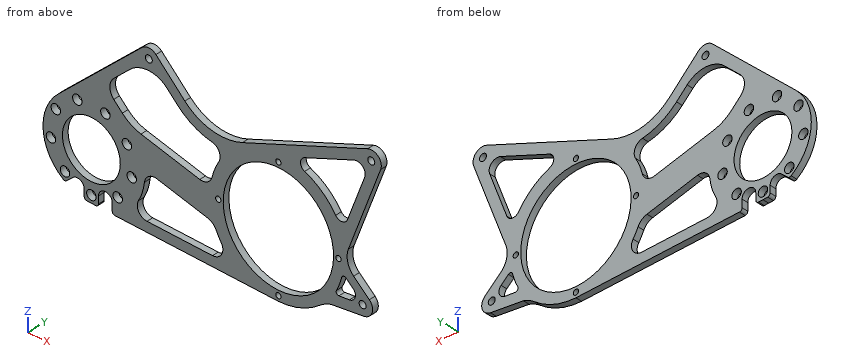
from build123d import *

# Parameters (mm, degrees)
MASTER_SKETCH_R       = 52.451
MASTER_SKETCH_R_2     = 9.525
MASTER_SKETCH_R_3     = 45.974
MASTER_SKETCH_R_4     = 27.4955
MASTER_SKETCH_R_5     = 6.5
BOSS_EXTRUDE2_DEPTH   = 3.048
F_5_0MM_DOWEL_HOLE1_D = 5
CIRPATTERN4_COUNT     = 4
M6_CLEARANCE_HOLE4_D  = 6.6
M8_CLEARANCE_HOLE1_D  = 9
CIRPATTERN3_COUNT     = 9
CUT_EXTRUDE2_DEPTH    = 284.854467488
CUT_EXTRUDE3_DEPTH    = 284.854467488
FILLET1_R             = 2.54


with BuildPart() as part:
    # Master Sketch → Boss-Extrude2 (new, symmetric)
    # profile 1 of 5: a face of its own
    with BuildSketch(Plane(origin=(0, 0, 0), x_dir=(1, 0, 0), z_dir=(0, 1, 0))):
        with BuildLine():
            ThreePointArc((-8.636, 127), (-36.396097826, 84.787887478), (-86.152093601, 93.552952189))
            Line((-86.152093601, 93.552952189), (-6.534964144, 18.470363023))
            ThreePointArc((-6.534964144, 18.470363023), (-3.773598517, 34.145603423), (9.525, 25.4))
            ThreePointArc((9.525, 25.4), (8.799952547, 21.754940307), (6.735192091, 18.664807909))
            Line((6.735192091, 18.664807909), (34.255961574, 46.185577392))
            ThreePointArc((34.255961574, 46.185577392), (59.945142207, 60.02346539), (89.010077776, 57.44457682))
            Line((89.010077776, 57.44457682), (207.987004211, 9.951947906))
            ThreePointArc((207.987004211, 9.951947906), (204.851852042, 25.601533276), (220.43444462, 22.148779315))
            Line((220.43444462, 22.148779315), (189.716874265, 103.891447497))
            ThreePointArc((189.716874265, 103.891447497), (189.0323732, 115.067445458), (194.744907427, 124.697524629))
            Line((194.744907427, 124.697524629), (209.652959731, 138.231042786))
            ThreePointArc((209.652959731, 138.231042786), (194.181291125, 142.373055798), (204.353700493, 154.744429565))
            Line((204.353700493, 154.744429565), (173.100049306, 158.387997533))
            ThreePointArc((173.100049306, 158.387997533), (167.382597042, 160.73155253), (162.227355528, 164.138163067))
            ThreePointArc((162.227355528, 164.138163067), (143.898999717, 174.415513345), (123.19, 177.9778))
            Line((123.19, 177.9778), (-54.61, 172.974))
            ThreePointArc((-54.61, 172.974), (-22.101472842, 159.508527158), (-8.636, 127))
        make_face()
        with Locations(Location((123.19, 116.0018, 0), (0, 0, 90))):
            Circle(MASTER_SKETCH_R, mode=Mode.SUBTRACT)
    # profile 2 of 5: a face of its own
    with BuildSketch(Plane(origin=(0, 0, 0), x_dir=(1, 0, 0), z_dir=(0, 1, 0))):
        with Locations((0, 25.4)):
            Circle(MASTER_SKETCH_R_2)
    # profile 3 of 5: a face of its own
    with BuildSketch(Plane(origin=(0, 0, 0), x_dir=(1, 0, 0), z_dir=(0, 1, 0))):
        with Locations((211.518208908, 18.79820239)):
            Circle(MASTER_SKETCH_R_2)
    # profile 4 of 5: a face of its own
    with BuildSketch(Plane(origin=(0, 0, 0), x_dir=(1, 0, 0), z_dir=(0, 1, 0))):
        with Locations((203.2507406, 145.283504427)):
            Circle(MASTER_SKETCH_R_2)
    # profile 5 of 5: a face of its own
    with BuildSketch(Plane(origin=(0, 0, 0), x_dir=(1, 0, 0), z_dir=(0, 1, 0))):
        with Locations((-54.61, 127)):
            Circle(MASTER_SKETCH_R_3)
        with Locations(Location((-54.61, 127, 0), (0, 0, 90))):
            Circle(MASTER_SKETCH_R_4, mode=Mode.SUBTRACT)
        with Locations(Location((-67.94878559, 163.648012211, 0), (0, 0, 90))):
            Circle(MASTER_SKETCH_R_5, mode=Mode.SUBTRACT)
        with Locations(Location((-41.27121441, 163.648012211, 0), (0, 0, 90))):
            Circle(MASTER_SKETCH_R_5, mode=Mode.SUBTRACT)
    extrude(amount=BOSS_EXTRUDE2_DEPTH, both=True)

    # Ø5.0mm Dowel Hole1 (through all)
    with Locations(Plane(origin=(0, 3.048, 0), x_dir=(1, 0, 0), z_dir=(0, 1, 0))):
        with Locations((123.19, 173.1518)):
            f_5_0mm_dowel_hole1 = Hole(F_5_0MM_DOWEL_HOLE1_D / 2)

    # CirPattern4: Ø5.0mm Dowel Hole1 ×4 about axis
    cirpattern4_axis = Axis((123.19, 0, -116.0018), (0, 1, 0))
    for i in range(1, CIRPATTERN4_COUNT):
        add(f_5_0mm_dowel_hole1.rotate(cirpattern4_axis, i * 360 / CIRPATTERN4_COUNT), mode=Mode.SUBTRACT)

    # M6 Clearance Hole4 (through all)
    with Locations(Plane(origin=(0, 3.048, 0), x_dir=(1, 0, 0), z_dir=(0, 1, 0))):
        with Locations((203.2507406, 145.283504427), (211.518208908, 18.79820239), (0, 25.4)):
            Hole(M6_CLEARANCE_HOLE4_D / 2)

    # M8 Clearance Hole1 (through all)
    with Locations(Plane(origin=(0, 3.048, 0), x_dir=(1, 0, 0), z_dir=(0, 1, 0))):
        with Locations((-54.61, 166)):
            m8_clearance_hole1 = Hole(M8_CLEARANCE_HOLE1_D / 2)

    # CirPattern3: M8 Clearance Hole1 ×9 about axis
    cirpattern3_axis = Axis((-54.61, 0, -127), (0, 1, 0))
    for i in range(1, CIRPATTERN3_COUNT):
        add(m8_clearance_hole1.rotate(cirpattern3_axis, i * 360 / CIRPATTERN3_COUNT), mode=Mode.SUBTRACT)

    # Topology 3 → Cut-Extrude2 (cut, through all)
    with BuildSketch(Plane(origin=(0, 3.048, 0), x_dir=(1, 0, 0), z_dir=(0, 1, 0))):
        with BuildLine():
            ThreePointArc((-17.945313453, 42.323250142), (-0.146601343, 35.405008389), (17.44176984, 42.84176984))
            Line((17.44176984, 42.84176984), (27.520769483, 52.920769483))
            ThreePointArc((27.520769483, 52.920769483), (42.409632623, 63.819008448), (59.896219631, 69.707058463))
            ThreePointArc((59.896219631, 69.707058463), (66.885503662, 75.024623751), (66.553177874, 83.800508404))
            ThreePointArc((66.553177874, 83.800508404), (62.745475764, 91.688999032), (60.030376503, 100.016970919))
            ThreePointArc((60.030376503, 100.016970919), (55.6852269, 105.854731176), (48.48636159, 106.920614917))
            Line((48.48636159, 106.920614917), (-7.457826773, 92.934567826))
            ThreePointArc((-7.457826773, 92.934567826), (-16.98904431, 89.126755018), (-25.157987823, 82.912906934))
            Line((-25.157987823, 82.912906934), (-33.299725858, 74.771168898))
            ThreePointArc((-33.299725858, 74.771168898), (-37.018106584, 65.604842248), (-33.032755262, 56.551396808))
            Line((-33.032755262, 56.551396808), (-17.945313453, 42.323250142))
        make_face()
        with BuildLine():
            ThreePointArc((64.098067009, 143.438932802), (66.306808777, 147.765857633), (68.831828447, 151.916170194))
            ThreePointArc((68.831828447, 151.916170194), (69.209050275, 161.796201373), (60.61677272, 166.688039353))
            Line((60.61677272, 166.688039353), (-1.663792567, 164.935286301))
            ThreePointArc((-1.663792567, 164.935286301), (-9.632748017, 160.197249287), (-9.798074059, 150.927626155))
            ThreePointArc((-9.798074059, 150.927626155), (-6.09260405, 142.056636088), (-4.12477238, 132.646396384))
            ThreePointArc((-4.12477238, 132.646396384), (-0.093621954, 125.882803807), (7.651359628, 124.464488392))
            Line((7.651359628, 124.464488392), (55.659374127, 136.466492017))
            ThreePointArc((55.659374127, 136.466492017), (60.668494681, 138.996854714), (64.098067009, 143.438932802))
        make_face()
        with BuildLine():
            ThreePointArc((148.153589294, 55.823132596), (164.735029841, 65.81551406), (177.648151764, 80.239214699))
            ThreePointArc((177.648151764, 80.239214699), (183.658143307, 83.064639882), (188.900120968, 78.987300553))
            Line((188.900120968, 78.987300553), (205.194131764, 35.627233252))
            ThreePointArc((205.194131764, 35.627233252), (203.319232726, 27.16564341), (194.821264757, 25.463207079))
            Line((194.821264757, 25.463207079), (148.232551201, 44.060262413))
            ThreePointArc((148.232551201, 44.060262413), (144.236830733, 49.915140022), (148.153589294, 55.823132596))
        make_face()
        with BuildLine():
            Line((187.419319265, 129.472737786), (194.351886978, 135.766117303))
            ThreePointArc((194.351886978, 135.766117303), (196.107471775, 142.477028469), (190.674704354, 146.790199554))
            Line((190.674704354, 146.790199554), (180.805871382, 147.712647003))
            ThreePointArc((180.805871382, 147.712647003), (178.552910329, 146.650002513), (178.398012452, 144.16383006))
            ThreePointArc((178.398012452, 144.16383006), (181.288513561, 137.579272003), (183.396839106, 130.704218196))
            ThreePointArc((183.396839106, 130.704218196), (185.057898436, 128.944655397), (187.419319265, 129.472737786))
        make_face()
    extrude(amount=-CUT_EXTRUDE2_DEPTH, mode=Mode.SUBTRACT)

    # Sketch29 → Cut-Extrude3 (cut, through all)
    with BuildSketch(Plane.XZ.offset(3.048)):
        with BuildLine():
            Line((-72.305646266, -158.824345033), (-79.713448931, -165.515263569))
            ThreePointArc((-79.713448931, -165.515263569), (-70.954498766, -169.970525201), (-61.44878559, -172.462508594))
            Line((-61.44878559, -172.462508594), (-61.44878559, -163.648012211))
            ThreePointArc((-61.44878559, -163.648012211), (-70.587952655, -169.588112984), (-72.305646266, -158.824345033))
        make_face()
        with BuildLine():
            Line((-47.77121441, -163.648012211), (-47.77121441, -173.166462966))
            Line((-47.77121441, -173.166462966), (-34.77121441, -173.532320109))
            Line((-34.77121441, -173.532320109), (-34.77121441, -163.648012211))
            ThreePointArc((-34.77121441, -163.648012211), (-41.27121441, -170.148012211), (-47.77121441, -163.648012211))
        make_face()
    extrude(amount=-CUT_EXTRUDE3_DEPTH, mode=Mode.SUBTRACT)

    # Fillet1
    fillet1_edges = [part.edges().sort_by_distance(p)[0] for p in [
        (-79.713448931, 0, -165.515263569),
        (-61.44878559, 0, -172.462508594),
        (-47.77121441, 0, -173.166462966),
        (-34.77121441, 0, -173.532320109),
    ]]
    fillet(fillet1_edges, radius=FILLET1_R)


solid = part.part
Work out the finished part from the listing and answer in its coordinate system (mm). Give positions to 0.01 mm unless a question says otherwise; leave off trailing zeros. Loops run counter-clockwise (first coordinate to the right, second up) from the corner with the lowest first, then second, coordinate; pieces in that order, holes last. Notation, with made-up numbers: (-7.75, 16.25) -> (8.25, 16.25) arc R23 ccw to (8.25, 49.25) -> close; hole circle Ø4 at (-13, 67). An arc over 180 degrees is marked (long way). Use a Markdown table: item, result. Add a question column.
1. Section B-B on y = 0 is taken. State how many separate pieces and enclosed holes the cut face has, and give its area (3 significant figures).
2. Flat-ended cylindrical pins translate along their axes: pin 1 Ø10.5 at (x, z) = (-93.02, -133.77) entering from +Y; pin 2 Ø1.8 at (y, z) = (1, -168.5) entering from +X; pin 3 Ø1 at (y, z) = (1.5, -61) entering from -X; pin 4 Ø3 at (x, y) = (85, 0.5) entering from -Z. Find the tip coordinate at first contact, or state that the pin passes through.
3. Section A-A on x = 136 is taken. Determine the outline of the cut face in (y, z), and give its area (3 significant figures).
4. Find the intervals of material crossed by probe 1 along X at (y, z) = (1.75, -80.5); probe 2 along Z at (x, y) = (-71.5, 0.5); probe 3 along X at (y, z) = (-2, -110), in increasing order.
Results below:
| question | item | result |
|---|---|---|
| 1 | separate pieces | 1 |
| 1 | enclosed holes | 22 |
| 1 | area | 16,500 mm^2 |
| 2 | pin 1 | stops at y = 3.05 |
| 2 | pin 2 | stops at x = 157.52 |
| 2 | pin 3 | stops at x = -52.16 |
| 2 | pin 4 | stops at z = -176.95 |
| 3 | outline | (-3.05, -176.64) -> (3.05, -176.64) -> (3.05, -166.86) -> (-3.05, -166.86) -> close; (-3.05, -65.14) -> (3.05, -65.14) -> (3.05, -38.69) -> (-3.05, -38.69) -> close |
| 3 | area | 221 mm^2 |
| 4 | probe 1 | x = -72.31 to -27.57, 67.69 to 84.58, 161.8 to 177.83, 188.08 to 198.51 |
| 4 | probe 2 | z = -158.2 to -148.7, -105.3 to -93.12, -87.59 to -79.74 |
| 4 | probe 3 | x = -97.33 to -92.13, -84.64 to -76.22, -33 to -24.58, -17.09 to 71.08, 175.3 to 188.51 |
